Geometry check sheet. Reference: the model listing, model coordinates, mm. Face numbers are marked on the shaded views. A direction names the side the tool comes from. Give positions to 0.01 mm unless a question says otherwise; leave off trailing zeros. Write each loop counter-clockwise with the first axis right and the second up, starting at its lowest first coordinate (ties: lowest second). Pieces come first, ordered by that corner, then holes. Notation, with made-up numbers: (-40, -22) -> (14, -22) arc R11 ccw to (14, -5) -> close; hole circle Ø5 at (-20, 39). An arc over 180 degrees is marked (long way). One line per item, written item: value.
from build123d import *

# Parameters (mm, degrees)
F1_DEPTH = 10
F2_SIZE  = 2


with BuildPart() as f1:
    # F0 (on Top) → F1 (new body)
    with BuildSketch(Plane.XY):
        Polygon((-15, 0), (0, 0), (15, 0), (15, 2.5), (6.5, 2.5), (6.5, 12.5), (2.5, 12.5), (2.5, 2.5), (0, 2.5), (-2.5, 2.5), (-2.5, 12.5), (-6.5, 12.5), (-6.5, 2.5), (-15, 2.5), align=None)
    extrude(amount=F1_DEPTH)

    # F2
    f2_edges = [f1.edges().sort_by_distance(p)[0] for p in [
        (-6.5, 12.5, 5),
        (-15, 2.5, 5),
        (6.5, 12.5, 5),
        (15, 2.5, 5),
    ]]
    chamfer(f2_edges, length=F2_SIZE)


solid = f1.part
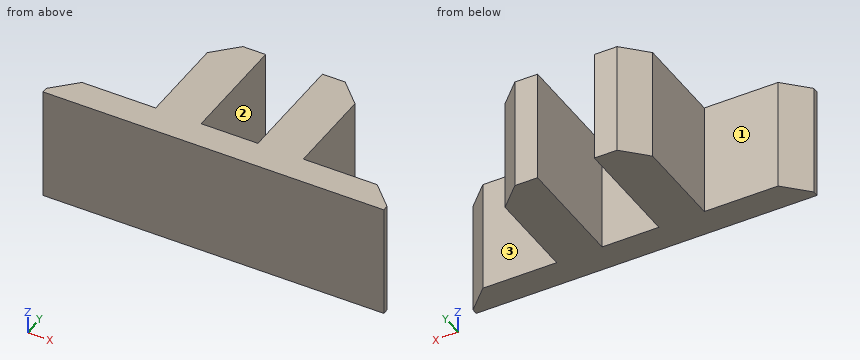
1) Depth check by flat-ended pin: pin 1 Ø5 at (x, z) = (8.5, 6) entering from +Y; pin 2 Ø3 at (x, z) = (-9, 3.5) entering from +Y; pin 3 Ø1 at (y, z) = (10.5, 8.5) entering from -X. Enter the tip coordinate at first touch or a pass-through.
Verdict:
pin 1: y = 11
pin 2: y = 2.5
pin 3: x = -6.5
2) Sectioned sample at C-C on x = -5. Record the cut outline in (y, z), plus the area to 3 significant figures.
Verdict:
outline: (0, 0) -> (12, 0) -> (12, 10) -> (0, 10) -> close
area: 120 mm^2
3) Sectioned sample at D-D on y = 1.75. Record the cut outline in (x, z).
Verdict:
outline: (-13.75, 0) -> (13.75, 0) -> (13.75, 10) -> (-13.75, 10) -> close
4) Sectioned sample at A-A on y = 8.75. Record the cut outline in (x, z), plus the area to 3 significant figures.
Verdict:
outline: (-6.5, 0) -> (-2.5, 0) -> (-2.5, 10) -> (-6.5, 10) -> close; (2.5, 0) -> (6.5, 0) -> (6.5, 10) -> (2.5, 10) -> close
area: 80.0 mm^2
5) Scan lines: probe 1 along X at (y, z) = (5, 4.25); probe 2 along Y at (x, z) = (-7.75, 7.25); probe 3 along X at (y, z) = (12.25, 3.25). Record each from-to range of solid material in increasing order.
Verdict:
probe 1: -6.5 to -2.5, 2.5 to 6.5
probe 2: 0 to 2.5
probe 3: -4.75 to -2.5, 2.5 to 4.75
6) Sectioned sample at B-B on z = 8.75. Record the cut outline in (x, y), plus the area to 3 significant figures.
Verdict:
outline: (-15, 0) -> (15, 0) -> (15, 0.5) -> (13, 2.5) -> (6.5, 2.5) -> (6.5, 10.5) -> (4.5, 12.5) -> (2.5, 12.5) -> (2.5, 2.5) -> (-2.5, 2.5) -> (-2.5, 12.5) -> (-4.5, 12.5) -> (-6.5, 10.5) -> (-6.5, 2.5) -> (-13, 2.5) -> (-15, 0.5) -> close
area: 147 mm^2
7) Tool access check on the marked faces 1, 2 and 3. Record the directions out of +Z, -Z, +X, -X, +Y, -Y that give a thin tool (end or side, any length) a straight path to the whole face; none if there is none.
Verdict:
face 1: +Z, -Z, -X, +Y
face 2: +Z, -Z, +Y
face 3: +Z, -Z, +X, +Y
